from build123d import *

# Parameters (mm, degrees)
F0_R     = 5.4
F1_DEPTH = 3
F1_TAPER = -3
F3_DEPTH = 3
F3_TAPER = -3
F5_DEPTH = 3
F5_TAPER = -3
F6_R     = 1


with BuildPart() as f1:
    # F0 (on Front) → F1 (new body)
    with BuildSketch(Plane.XZ):
        Circle(F0_R)
        with BuildLine():
            ThreePointArc((1.525, 2.1057955741), (2.3157072354, 1.1821590418), (2.6, 0))
            ThreePointArc((2.6, 0), (2.3157072354, -1.1821590418), (1.525, -2.1057955741))
            ThreePointArc((1.525, -2.1057955741), (0, -2.6), (-1.525, -2.1057955741))
            ThreePointArc((-1.525, -2.1057955741), (-2.6, 0), (-1.525, 2.1057955741))
            ThreePointArc((-1.525, 2.1057955741), (0, 2.6), (1.525, 2.1057955741))
        make_face(mode=Mode.SUBTRACT)
        with BuildLine():
            ThreePointArc((1.525, -2.1057955741), (2.3157072354, -1.1821590418), (2.6, 0))
            ThreePointArc((2.6, 0), (2.3157072354, 1.1821590418), (1.525, 2.1057955741))
            Line((1.525, 2.1057955741), (1.525, -2.1057955741))
        make_face()
        with BuildLine():
            Line((-1.525, -2.1057955741), (-1.525, 2.1057955741))
            ThreePointArc((-1.525, 2.1057955741), (-2.6, 0), (-1.525, -2.1057955741))
        make_face()
    extrude(amount=F1_DEPTH, taper=F1_TAPER)

    # F2 (on face) → F3 (join)
    with BuildSketch(Plane.XZ.offset(3)):
        Polygon((3.2222269322, 35), (0, 35), (-3.2222269322, 35), (-2, 0), (0, 0), (2, 0), align=None)
    extrude(amount=-F3_DEPTH, taper=F3_TAPER)

    # F4 (on face) → F5 (join)
    with BuildSketch(Plane.XZ.offset(3)):
        Polygon((0, 47.5), (-7.5, 35), (-3.2222269322, 35), (3.2222269322, 35), (7.5, 35), align=None)
    extrude(amount=-F5_DEPTH, taper=F5_TAPER)

    # F6
    f6_edges = [f1.edges().sort_by_distance(p)[0] for p in [
        (0, -1.5, 47.652794),
        (-7.638843, -1.5, 34.921388),
        (7.638843, -1.5, 34.921388),
    ]]
    fillet(f6_edges, radius=F6_R)


solid = f1.part
Geometry check sheet. Reference: the model listing, model coordinates, mm. Give positions to 0.01 mm unless a question says otherwise; leave off trailing zeros.
1) Draft check along Z on faces 1 (the flat face through (-1, -3, 21)), 2 (the conical face through (-0.21, -1.19, -5.46)). Enter one of: released by +Z, released by -Z, zero draft, split by the parting line, or undercut.
Results are:
face 1: zero draft
face 2: undercut
2) Material ranges on probe 1 along Z at (x, y) = (-0.5, -1.55); probe 2 along Z at (x, y) = (-4, -2.35); probe 3 along X at (y, z) = (-1.3, 38), recorded low to high.
Results are:
probe 1: z = -5.46 to -2.47, -0.08 to 46.57
probe 2: z = -3.81 to 3.81, 34.97 to 40.9
probe 3: x = -5.8 to 5.8
3) Gauge pin test, flat end, axial feed: pin 1 (1 mm diameter, centred on x = 2, y = -1.5, fed in from +Z). Record the tip position at first contact, or that the pin passes through.
Results are:
pin 1: stops at z = 45.15
